from build123d import *

# Parameters (mm, degrees)
BOSS_EXTRU_1_DEPTH      = 15
CONG_1_R                = 2
ENL_V_MAT_EXTRU_1_REACH = 4
ESQUISSE2_R             = 2.5
ENL_V_MAT_EXTRU_2_REACH = 4
ESQUISSE3_R             = 2.5


with BuildPart() as part:
    # Esquisse1 → Boss.-Extru.1 (new body, symmetric)
    with BuildSketch(Plane(origin=(0, 0, 0), x_dir=(0, 0, -1), z_dir=(1, 0, 0))):
        Polygon((0, 0), (0, 50), (2, 50), (2, 2), (55, 2), (55, 0), align=None)
    extrude(amount=BOSS_EXTRU_1_DEPTH, both=True)

    # Congé1
    cong_1_edges = [part.edges().sort_by_distance(p)[0] for p in [
        (0, 0, 0),
        (0, 2, -2),
    ]]
    fillet(cong_1_edges, radius=CONG_1_R)

    # Esquisse2 → Enlèv. mat.-Extru.1 (cut, up to next)
    with BuildSketch(Plane(origin=(0, 2, 0), x_dir=(1, 0, 0), z_dir=(0, 1, 0)), mode=Mode.PRIVATE) as enl_v_mat_extru_1_sk1:
        with BuildLine():
            Line((4.25, 24.25), (4.25, 45.75))
            ThreePointArc((4.25, 45.75), (0, 50), (-4.25, 45.75))
            Line((-4.25, 45.75), (-4.25, 24.25))
            ThreePointArc((-4.25, 24.25), (0, 20), (4.25, 24.25))
        make_face()
    enl_v_mat_extru_1_tool1 = extrude(enl_v_mat_extru_1_sk1.sketch, amount=-ENL_V_MAT_EXTRU_1_REACH, mode=Mode.PRIVATE) & part.part
    add(enl_v_mat_extru_1_tool1.solids().sort_by_distance((0, 2, -35))[0], mode=Mode.SUBTRACT)
    # Esquisse2 → Enlèv. mat.-Extru.1 (cut, up to next)
    with BuildSketch(Plane(origin=(0, 2, 0), x_dir=(1, 0, 0), z_dir=(0, 1, 0)), mode=Mode.PRIVATE) as enl_v_mat_extru_1_sk2:
        with Locations((-9.5, 25)):
            Circle(ESQUISSE2_R)
    enl_v_mat_extru_1_tool2 = extrude(enl_v_mat_extru_1_sk2.sketch, amount=-ENL_V_MAT_EXTRU_1_REACH, mode=Mode.PRIVATE) & part.part
    add(enl_v_mat_extru_1_tool2.solids().sort_by_distance((-9.5, 2, -25))[0], mode=Mode.SUBTRACT)
    # Esquisse2 → Enlèv. mat.-Extru.1 (cut, up to next)
    with BuildSketch(Plane(origin=(0, 2, 0), x_dir=(1, 0, 0), z_dir=(0, 1, 0)), mode=Mode.PRIVATE) as enl_v_mat_extru_1_sk3:
        with Locations((-9.5, 45)):
            Circle(ESQUISSE2_R)
    enl_v_mat_extru_1_tool3 = extrude(enl_v_mat_extru_1_sk3.sketch, amount=-ENL_V_MAT_EXTRU_1_REACH, mode=Mode.PRIVATE) & part.part
    add(enl_v_mat_extru_1_tool3.solids().sort_by_distance((-9.5, 2, -45))[0], mode=Mode.SUBTRACT)
    # Esquisse2 → Enlèv. mat.-Extru.1 (cut, up to next)
    with BuildSketch(Plane(origin=(0, 2, 0), x_dir=(1, 0, 0), z_dir=(0, 1, 0)), mode=Mode.PRIVATE) as enl_v_mat_extru_1_sk4:
        with Locations((9.5, 45)):
            Circle(ESQUISSE2_R)
    enl_v_mat_extru_1_tool4 = extrude(enl_v_mat_extru_1_sk4.sketch, amount=-ENL_V_MAT_EXTRU_1_REACH, mode=Mode.PRIVATE) & part.part
    add(enl_v_mat_extru_1_tool4.solids().sort_by_distance((9.5, 2, -45))[0], mode=Mode.SUBTRACT)
    # Esquisse2 → Enlèv. mat.-Extru.1 (cut, up to next)
    with BuildSketch(Plane(origin=(0, 2, 0), x_dir=(1, 0, 0), z_dir=(0, 1, 0)), mode=Mode.PRIVATE) as enl_v_mat_extru_1_sk5:
        with Locations((9.5, 25)):
            Circle(ESQUISSE2_R)
    enl_v_mat_extru_1_tool5 = extrude(enl_v_mat_extru_1_sk5.sketch, amount=-ENL_V_MAT_EXTRU_1_REACH, mode=Mode.PRIVATE) & part.part
    add(enl_v_mat_extru_1_tool5.solids().sort_by_distance((9.5, 2, -25))[0], mode=Mode.SUBTRACT)

    # Esquisse3 → Enlèv. mat.-Extru.2 (cut, up to next)
    with BuildSketch(Plane(origin=(0, 0, -2), x_dir=(-1, 0, 0), z_dir=(0, 0, -1)), mode=Mode.PRIVATE) as enl_v_mat_extru_2_sk1:
        with BuildLine():
            Line((-4.25, 40), (-4.25, 18.5))
            ThreePointArc((-4.25, 18.5), (0, 14.25), (4.25, 18.5))
            Line((4.25, 18.5), (4.25, 40))
            ThreePointArc((4.25, 40), (0, 44.25), (-4.25, 40))
        make_face()
    enl_v_mat_extru_2_tool1 = extrude(enl_v_mat_extru_2_sk1.sketch, amount=-ENL_V_MAT_EXTRU_2_REACH, mode=Mode.PRIVATE) & part.part
    add(enl_v_mat_extru_2_tool1.solids().sort_by_distance((0, 29.25, -2))[0], mode=Mode.SUBTRACT)
    # Esquisse3 → Enlèv. mat.-Extru.2 (cut, up to next)
    with BuildSketch(Plane(origin=(0, 0, -2), x_dir=(-1, 0, 0), z_dir=(0, 0, -1)), mode=Mode.PRIVATE) as enl_v_mat_extru_2_sk2:
        with Locations((-9.5, 40)):
            Circle(ESQUISSE3_R)
    enl_v_mat_extru_2_tool2 = extrude(enl_v_mat_extru_2_sk2.sketch, amount=-ENL_V_MAT_EXTRU_2_REACH, mode=Mode.PRIVATE) & part.part
    add(enl_v_mat_extru_2_tool2.solids().sort_by_distance((9.5, 40, -2))[0], mode=Mode.SUBTRACT)
    # Esquisse3 → Enlèv. mat.-Extru.2 (cut, up to next)
    with BuildSketch(Plane(origin=(0, 0, -2), x_dir=(-1, 0, 0), z_dir=(0, 0, -1)), mode=Mode.PRIVATE) as enl_v_mat_extru_2_sk3:
        with Locations((9.5, 40)):
            Circle(ESQUISSE3_R)
    enl_v_mat_extru_2_tool3 = extrude(enl_v_mat_extru_2_sk3.sketch, amount=-ENL_V_MAT_EXTRU_2_REACH, mode=Mode.PRIVATE) & part.part
    add(enl_v_mat_extru_2_tool3.solids().sort_by_distance((-9.5, 40, -2))[0], mode=Mode.SUBTRACT)
    # Esquisse3 → Enlèv. mat.-Extru.2 (cut, up to next)
    with BuildSketch(Plane(origin=(0, 0, -2), x_dir=(-1, 0, 0), z_dir=(0, 0, -1)), mode=Mode.PRIVATE) as enl_v_mat_extru_2_sk4:
        with Locations((9.5, 18.5)):
            Circle(ESQUISSE3_R)
    enl_v_mat_extru_2_tool4 = extrude(enl_v_mat_extru_2_sk4.sketch, amount=-ENL_V_MAT_EXTRU_2_REACH, mode=Mode.PRIVATE) & part.part
    add(enl_v_mat_extru_2_tool4.solids().sort_by_distance((-9.5, 18.5, -2))[0], mode=Mode.SUBTRACT)
    # Esquisse3 → Enlèv. mat.-Extru.2 (cut, up to next)
    with BuildSketch(Plane(origin=(0, 0, -2), x_dir=(-1, 0, 0), z_dir=(0, 0, -1)), mode=Mode.PRIVATE) as enl_v_mat_extru_2_sk5:
        with Locations((-9.5, 18.5)):
            Circle(ESQUISSE3_R)
    enl_v_mat_extru_2_tool5 = extrude(enl_v_mat_extru_2_sk5.sketch, amount=-ENL_V_MAT_EXTRU_2_REACH, mode=Mode.PRIVATE) & part.part
    add(enl_v_mat_extru_2_tool5.solids().sort_by_distance((9.5, 18.5, -2))[0], mode=Mode.SUBTRACT)


solid = part.part
Design review of the part built by this model. Coordinates are the model's own, in mm. A direction names the side the tool comes from. Round coordinates to 2 decimals unless told otherwise and drop trailing zeros. Write each loop counter-clockwise with the first axis right and the second up, starting at its lowest first coordinate (ties: lowest second). Pieces come first, ordered by that corner, then holes.
Item 1: For pin 1 Ø8 at (x, y) = (9.5, 18.5) entering from +Z; pin 2 Ø8 at (x, y) = (-9.5, 40) entering from -Z; pin 3 Ø3 at (x, z) = (10, -44) entering from +Y, all flat-tipped, find the tip position at first contact; note any pin that passes through.
Item 2: Consider section C-C on y = 26. Give the boundary of the cut face in (x, z).
Item 3: Wall thickness on L1, parallel to Z at x = 9.5, y = 0.9; L2, parallel to Y at x = -9.5, z = -1.3; L3, parallel to Y at x = 9.5, z = -0.55: over which ranges is each line inside the solid? List them lowest first.
Item 4: Consider section D-D on x = -9.5. Give the boundary of the cut face in (y, z), and give its area (3 significant figures).
Item 5: Draft analysis for pull direction Y (two halves, no side actions). For faces 5 (the cylindrical face through (0, 1, -50)), 6 (the cylindrical face through (0.21, 0.6, -0.57)), 7 (the cylindrical face through (-9.17, 20.98, -1.01)), state which applies: released by +Y, released by -Y, zero draft, split by the parting line, or undercut.
Item 6: For faces 1 (the flat face through (0, 50, -1)), 2 (the flat face through (-4.25, 29, -1)), 3 (the flat face through (4.25, 1, -35)), 4 (the flat face through (7, 27, -2)), list the 3-axis set-ups (+Z, -Z, +X, -X, +Y, -Y) from which the entire face can be reached by the end or side of a thin tool; tool diameter is ignored.
Item 7: Consider section B-B on x = 0. Give the boundary of the cut face in (y, z).
Item 8: Consider section A-A on z = -25. Give the boundary of the cut face in (x, y), and give its area (3 significant figures).
Check values:
1. pin 1: stops at z = 0
1. pin 2: stops at z = -2
1. pin 3: stops at y = 2
2. outline: (-15, -2) - (-4.25, -2) - (-4.25, 0) - (-15, 0) - close; (4.25, -2) - (15, -2) - (15, 0) - (4.25, 0) - close
3. L1: z = -55 to -47.5, -42.5 to -27.5, -22.5 to -0.33
3. L2: y = 0.13 to 16, 21 to 37.5, 42.5 to 50
3. L3: y = 0.62 to 16, 21 to 37.5, 42.5 to 50
4. outline: (0, -55) - (2, -55) - (2, -47.5) - (0, -47.5) - close; (0, -42.5) - (2, -42.5) - (2, -27.5) - (0, -27.5) - close; (0, -22.5) - (2, -22.5) - (2, -4) arc R2 cw to (4, -2) - (16, -2) - (16, 0) - (2, 0) arc R2 ccw to (0, -2) - close; (21, -2) - (37.5, -2) - (37.5, 0) - (21, 0) - close; (42.5, -2) - (50, -2) - (50, 0) - (42.5, 0) - close
4. area: 166 mm2
5. face 5: zero draft
5. face 6: released by -Y
5. face 7: undercut
6. face 1: +Z, -Z, +X, -X, +Y
6. face 2: +Z, -Z
6. face 3: +Y, -Y
6. face 4: -Z, +X, -X, +Y
7. outline: (0, -55) - (2, -55) - (2, -50) - (0, -50) - close; (0, -20) - (2, -20) - (2, -4) arc R2 cw to (4, -2) - (14.25, -2) - (14.25, 0) - (2, 0) arc R2 ccw to (0, -2) - close; (44.25, -2) - (50, -2) - (50, 0) - (44.25, 0) - close
8. outline: (-15, 0) - (-12, 0) - (-12, 2) - (-15, 2) - close; (-7, 0) - (-4.25, 0) - (-4.25, 2) - (-7, 2) - close; (4.25, 0) - (7, 0) - (7, 2) - (4.25, 2) - close; (12, 0) - (15, 0) - (15, 2) - (12, 2) - close
8. area: 23.0 mm2
